from build123d import *

# Parameters (mm, degrees)
CROQUIS1_W              = 13.5
CROQUIS1_H              = 10.5
CROQUIS1_R              = 1.7
CROQUIS1_W_2            = 3
CROQUIS1_H_2            = 6.5
SALIENTE_EXTRUIR1_DEPTH = 7.1
CROQUIS2_W              = 5
CROQUIS2_H              = 8.5
CORTAR_EXTRUIR1_DEPTH   = 5.1


with BuildPart() as part:
    # Croquis1 → Saliente-Extruir1 (new body)
    with BuildSketch(Plane(origin=(0, 0, 0), x_dir=(1, 0, 0), z_dir=(0, 1, 0))):
        with Locations((14.85529294, -1.794299578)):
            Rectangle(CROQUIS1_W, CROQUIS1_H)
        with Locations((18.10529294, -1.913201206)):
            Circle(CROQUIS1_R, mode=Mode.SUBTRACT)
        with Locations((12.10529294, -1.794299578)):
            Rectangle(CROQUIS1_W_2, CROQUIS1_H_2, mode=Mode.SUBTRACT)
    extrude(amount=SALIENTE_EXTRUIR1_DEPTH)

    # Croquis2 → Cortar-Extruir1 (cut)
    with BuildSketch(Plane(origin=(0, 7.1, 0), x_dir=(1, 0, 0), z_dir=(0, 1, 0))):
        with Locations((12.10529294, -1.794299578)):
            Rectangle(CROQUIS2_W, CROQUIS2_H)
    extrude(amount=-CORTAR_EXTRUIR1_DEPTH, mode=Mode.SUBTRACT)


solid = part.part
The model under review builds one solid part; all positions refer to its coordinate system, in mm. A direction names the side the tool comes from. Give positions to 0.01 mm unless a question says otherwise; leave off trailing zeros. Loops run counter-clockwise (first coordinate to the right, second up) from the corner with the lowest first, then second, coordinate; pieces in that order, holes last. Notation, with made-up numbers: (71.25, 1.5) -> (107.25, 1.5) arc R16 cw to (107.25, 29.5) -> close; hole circle Ø8 at (10.25, 80). An arc over 180 degrees is marked (long way). Answer as a JSON object with one key per item and string values. Group by question number.
Q1. Take a section at C-C (z = 1). Write out the cut boundary in (x, y).
Q2. Tool access review of faces 5 (the flat face through (15, 0, 2)), 6 (the flat face through (12, 1, 5.044)), 7 (the flat face through (12, 5, -2.456)): name each direction out of +Z, -Z, +X, -X, +Y, -Y from which nothing blocks a thin tool from reaching the whole face with its end or side.
Q3. Take a section at B-B (z = -1.75). Write out the cut boundary in (x, y).
Q4. Take a section at D-D (y = 1). Write out the cut boundary in (x, z), plus the area to 3 significant figures.
Q5. Wall thickness on line 1 along X through (y, z) = (4.5, -2.25); line 2 along Z through (x, y) = (14.5, 5.25); line 3 along X through (y, z) = (1, 2.75): over which ranges is each line inside the solid? List them lowest first.
Q6. Insertion check: pin 1 (1 mm diameter, centred on x = 14, z = 5, fed in from +Y); pin 2 (5.5 mm diameter, centred on x = 18.11, z = 1.91, fed in from -Y). Each pin has a flat end and moves straight along its axis. Give the tip position at first contact, or say it passes through.
Q7. Take a section at A-A (x = 18.75). Write out the cut boundary in (y, z).
Q8. Draft analysis for pull direction Z (two halves, no side actions). For faces 1 (the flat face through (15, 4, 7.044)), 2 (the flat face through (12, 5, 6.044)), 3 (the flat face through (9.605, 5, 2)), 4 (the flat face through (16, 7.1, 2)), state which applies: pulls with the +Z half, pulls with the -Z half, needs draft (parallel to the pull), parting line crosses it, or undercut.
Answer below:
{
 "1": {"outline": "(8.11, 0) -> (10.61, 0) -> (10.61, 2) -> (9.61, 2) -> (9.61, 7.1) -> (8.11, 7.1) -> close; (13.61, 0) -> (16.67, 0) -> (16.67, 7.1) -> (14.61, 7.1) -> (14.61, 2) -> (13.61, 2) -> close; (19.54, 0) -> (21.61, 0) -> (21.61, 7.1) -> (19.54, 7.1) -> close"},
 "2": {"face 5": "+Z, -Z, +X, -X, -Y", "face 6": "+Y, -Y", "face 7": "+Y"},
 "3": {"outline": "(8.11, 0) -> (21.61, 0) -> (21.61, 7.1) -> (14.61, 7.1) -> (14.61, 2) -> (9.61, 2) -> (9.61, 7.1) -> (8.11, 7.1) -> close"},
 "4": {"outline": "(8.11, -3.46) -> (21.61, -3.46) -> (21.61, 7.04) -> (8.11, 7.04) -> close; hole (10.61, -1.46) -> (13.61, -1.46) -> (13.61, 5.04) -> (10.61, 5.04) -> close; hole circle Ø3.4 at (18.11, 1.91)", "area": "113 mm2"},
 "5": {"line 1": "x = 8.11 to 9.61, 14.61 to 21.61", "line 2": "z = -3.46 to -2.46, 6.04 to 7.04", "line 3": "x = 8.11 to 10.61, 13.61 to 16.63, 19.59 to 21.61"},
 "6": {"pin 1": "stops at y = 2", "pin 2": "stops at y = 0"},
 "7": {"outline": "(0, -3.46) -> (7.1, -3.46) -> (7.1, 0.34) -> (0, 0.34) -> close; (0, 3.49) -> (7.1, 3.49) -> (7.1, 7.04) -> (0, 7.04) -> close"},
 "8": {"face 1": "pulls with the +Z half", "face 2": "undercut", "face 3": "undercut", "face 4": "needs draft"}
}
